Check sheet for the modelled part. Datum: model origin and axes. Units: mm. A direction names the side the tool comes from. Give positions to 0.01 mm unless a question says otherwise; leave off trailing zeros. Loops run counter-clockwise (first coordinate to the right, second up) from the corner with the lowest first, then second, coordinate; pieces in that order, holes last. Notation, with made-up numbers: (82.25, 4) - (140.25, 4) arc R19 cw to (140.25, 20) - close; hole circle Ø3 at (-11.5, 43). An arc over 180 degrees is marked (long way). Use one line per item in the form item = value.
from build123d import *

# Parameters (mm, degrees)
F0_W      = 152.4
F0_H      = 76.2
F1_DEPTH  = 76.2
F2_R      = 36.7926146906
F3_W      = 69.3711452186
F3_H      = 30.6049170904
F4_DEPTH  = 69.342
F5_W      = 34.1026219539
F5_H      = 34.6188608486
F5_H_2    = 5.6047446165
F5_W_2    = 11.9504891336
F5_H_3    = 34.3273866851
F5_H_4    = 6.1876957375
F5_W_3    = 11.3675482571
F6_DEPTH  = 65.024
F7_W      = 65.5819708481
F7_H      = 16.0311469808
F8_DEPTH  = 83.82
F9_DEPTH  = 66.548
F7_W_2    = 68.2052476332
F7_H_2    = 8.5985241458
F7_W_3    = 67.330816295
F7_H_3    = 16.6140981019
F10_DEPTH = 100.076
F11_DEPTH = 87.63


with BuildPart() as f1:
    # F0 (on Top) → F1 (new body)
    with BuildSketch(Plane.XY):
        with Locations((-0.1249154925, 1.811310178)):
            Rectangle(F0_W, F0_H)
    extrude(amount=F1_DEPTH)

    # F2
    f2_edges = [f1.edges().sort_by_distance(p)[0] for p in [
        (-0.124915, -36.28869, 76.2),
    ]]
    fillet(f2_edges, radius=F2_R)

    # F3 (on face) → F4 (cut)
    with BuildSketch(Plane.XY.offset(76.2)):
        with Locations((-38.8286877424, 20.6947533879)):
            Rectangle(F3_W, F3_H)
    extrude(amount=-F4_DEPTH, mode=Mode.SUBTRACT)

    # F5 (on face) → F6 (cut)
    with BuildSketch(Plane.XY.offset(76.2)):
        with Locations((21.6524621937, 17.8133552929)):
            Rectangle(F5_W, F5_H)
        with Locations((21.6524621937, -2.2984474396)):
            Rectangle(F5_W, F5_H_2)
        with Locations((50.2170491964, 17.6676182112)):
            Rectangle(F5_W_2, F5_H_3)
        with Locations((50.2170491964, -2.5899230002)):
            Rectangle(F5_W_2, F5_H_4)
        with Locations((66.8311472982, 17.6676182112)):
            Rectangle(F5_W_3, F5_H_3)
        with Locations((66.8311472982, -2.5899230002)):
            Rectangle(F5_W_3, F5_H_4)
    extrude(amount=-F6_DEPTH, mode=Mode.SUBTRACT)

    # F7 (on Top) → F8 (join)
    with BuildSketch(Plane.XY):
        with Locations((38.8495135121, -23.3180331998)):
            Rectangle(F7_W, F7_H)
    extrude(amount=F8_DEPTH)

    # F9 (cut): a face of the model
    f9_faces = [f1.faces().sort_by_distance(p)[0] for p in [
        (38.8495135121, -23.3180331998, 83.82),
    ]]
    extrude(f9_faces, amount=-F9_DEPTH, mode=Mode.SUBTRACT)

    # F7 (on Top) → F10 (join)
    with BuildSketch(Plane.XY):
        with Locations((-38.5372140445, -4.2992620729)):
            Rectangle(F7_W_2, F7_H_2)
        with Locations((-38.3914739359, -23.0265576392)):
            Rectangle(F7_W_3, F7_H_3)
        with Locations((38.8495135121, -23.3180331998)):
            Rectangle(F7_W, F7_H)
    extrude(amount=F10_DEPTH)

    # F11 (cut): faces of the model
    f11_faces = [f1.faces().sort_by_distance(p)[0] for p in [
        (-38.3914739359, -23.0265576392, 100.076),
        (-38.5372140445, -4.2992620729, 100.076),
        (38.8495135121, -23.3180331998, 100.076),
    ]]
    extrude(f11_faces, amount=-F11_DEPTH, mode=Mode.SUBTRACT)


solid = f1.part
Item 1: Thickness scan on L1, parallel to X at y = -24, z = 18.5; L2, parallel to X at y = -1.5, z = 63.5; L3, parallel to X at y = 33, z = 13. Record the ranges inside material, lowest first.
Answer block:
L1 = -76.32 to -72.06, -4.73 to 6.06, 71.64 to 76.08
L2 = -76.32 to -72.64, -4.43 to 4.6, 38.7 to 44.24, 56.19 to 61.15, 72.51 to 76.08
L3 = -76.32 to -73.51, -4.14 to 4.6, 38.7 to 44.24, 56.19 to 61.15, 72.51 to 76.08
Item 2: Section check A-A on z = 32. Give the number of separate pieces and of enclosed holes in the cut face, then the cut area to 3 significant figures.
Answer block:
separate_pieces = 1
enclosed_holes = 7
area = 4,420 mm2
Item 3: Section check D-D on x = 51. Record the boundary of the cut face in (y, z).
Answer block:
outline = (-36.29, 0) - (39.91, 0) - (39.91, 76.2) - (34.83, 76.2) - (34.83, 11.18) - (-5.68, 11.18) - (-5.68, 75.68) arc R36.79 ccw to (-15.3, 72.63) - (-15.3, 12.45) - (-31.33, 12.45) - (-31.33, 57.85) arc R36.79 ccw to (-36.29, 39.41) - close
Item 4: Section check B-B on x = 12. Record the boundary of the cut face in (y, z), then the cut area to 3 significant figures.
Answer block:
outline = (-36.29, 0) - (39.91, 0) - (39.91, 76.2) - (35.12, 76.2) - (35.12, 11.18) - (-5.1, 11.18) - (-5.1, 75.77) arc R36.79 ccw to (-15.3, 72.63) - (-15.3, 12.45) - (-31.33, 12.45) - (-31.33, 57.85) arc R36.79 ccw to (-36.29, 39.41) - close
area = 2,030 mm2
Item 5: Gauge pin test, flat ends, axial feed: P1, Ø5, axis at x = 39, y = -25.5, coming from the +Z side; P2, Ø6, axis at x = 34.5, y = 20, coming from the +Z side. Record the tip position at first contact, or that the pin passes through.
Answer block:
P1 = 12.45
P2 = 11.18
Item 6: Section check C-C on y = 30. Record the boundary of the cut face in (x, z).
Answer block:
outline = (-76.32, 0) - (76.08, 0) - (76.08, 76.2) - (72.51, 76.2) - (72.51, 11.18) - (61.15, 11.18) - (61.15, 76.2) - (56.19, 76.2) - (56.19, 11.18) - (44.24, 11.18) - (44.24, 76.2) - (38.7, 76.2) - (38.7, 11.18) - (4.6, 11.18) - (4.6, 76.2) - (-4.14, 76.2) - (-4.14, 6.86) - (-73.51, 6.86) - (-73.51, 76.2) - (-76.32, 76.2) - close
Item 7: Access from +Z, -Z, +X, -X, +Y, -Y to the whole of each face (thin tool, end or side, straight path). Record for faces 1 (the face through (0.942, -29.865, 60.178)), 2 (the face through (21, 15, 11.176)).
Answer block:
face_1 = +Z, +X, -X, -Y
face_2 = +Z
Item 8: Mould release check, pull along X, two halves, no side actions. Record for faces 3 (the face through (50, 34.831, 44)), 4 (the face through (76.075, 1, 38)), 5 (the face through (-1, 2, 0)): released by +X, released by -X, zero draft, split by the parting line, or undercut.
Answer block:
face_3 = undercut
face_4 = released by +X
face_5 = zero draft
